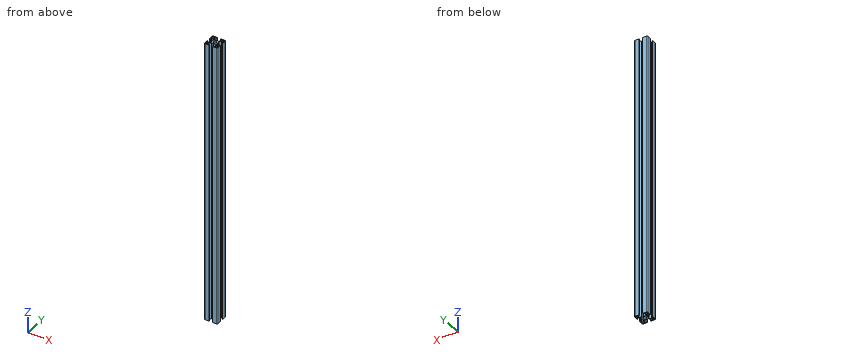
Autodesk Inventor part; units mm, degrees
ref_plane "C1_XY" through (0, 0, 0) normal (0, 0, 1) x (1, 0, 0)
ref_plane "C1_YZ" through (0, 0, 0) normal (1, 0, 0) x (0, 1, 0)
ref_plane "C1_ZX" through (0, 0, 0) normal (0, 1, 0) x (0, 0, 1)
sketch "Sketch_1" plane through (0, 0, 0) normal (0, 0, 1) x (1, 0, 0)
  line L0 (-15, 4) -> (-13, 4)
  line L1 (-13, 4) -> (-13, 8.25)
  line L2 (-13, 8.25) -> (-9.6642, 8.25)
  line L3 (-9.6642, 8.25) -> (-6, 4.5858)
  line L4 (-6, 4.5858) -> (-6, 0.5196)
  line L5 (-6, 0.5196) -> (-5.7, 0)
  line L6 (-5.7, 0) -> (-6, -0.5196)
  line L7 (-6, -0.5196) -> (-6, -4.5858)
  line L8 (-6, -4.5858) -> (-9.6642, -8.25)
  line L9 (-9.6642, -8.25) -> (-13, -8.25)
  line L10 (-13, -8.25) -> (-13, -4)
  line L11 (-13, -4) -> (-15, -4)
  line L12 (-15, -4) -> (-15, -13)
  arc A0 (-15, -13) -> (-13, -15) centre (-13, -13) ccw
  line L13 (-13, -15) -> (-4, -15)
  line L14 (-4, -15) -> (-4, -13)
  line L15 (-4, -13) -> (-8.25, -13)
  line L16 (-8.25, -13) -> (-8.25, -9.6642)
  line L17 (-8.25, -9.6642) -> (-4.5858, -6)
  line L18 (-4.5858, -6) -> (-0.5196, -6)
  line L19 (-0.5196, -6) -> (0, -5.7)
  line L20 (0, -5.7) -> (0.5196, -6)
  line L21 (0.5196, -6) -> (4.5858, -6)
  line L22 (4.5858, -6) -> (8.25, -9.6642)
  line L23 (8.25, -9.6642) -> (8.25, -13)
  line L24 (8.25, -13) -> (4, -13)
  line L25 (4, -13) -> (4, -15)
  line L26 (4, -15) -> (13, -15)
  arc A1 (13, -15) -> (15, -13) centre (13, -13) ccw
  line L27 (15, -13) -> (15, -4)
  line L28 (15, -4) -> (13, -4)
  line L29 (13, -4) -> (13, -8.25)
  line L30 (13, -8.25) -> (9.6642, -8.25)
  line L31 (9.6642, -8.25) -> (6, -4.5858)
  line L32 (6, -4.5858) -> (6, -0.5196)
  line L33 (6, -0.5196) -> (5.7, 0)
  line L34 (5.7, 0) -> (6, 0.5196)
  line L35 (6, 0.5196) -> (6, 4.5858)
  line L36 (6, 4.5858) -> (9.6642, 8.25)
  line L37 (9.6642, 8.25) -> (13, 8.25)
  line L38 (13, 8.25) -> (13, 4)
  line L39 (13, 4) -> (15, 4)
  line L40 (15, 4) -> (15, 13)
  arc A2 (15, 13) -> (13, 15) centre (13, 13) ccw
  line L41 (13, 15) -> (4, 15)
  line L42 (4, 15) -> (4, 13)
  line L43 (4, 13) -> (8.25, 13)
  line L44 (8.25, 13) -> (8.25, 9.6642)
  line L45 (8.25, 9.6642) -> (4.5858, 6)
  line L46 (4.5858, 6) -> (0.5196, 6)
  line L47 (0.5196, 6) -> (0, 5.7)
  line L48 (0, 5.7) -> (-0.5196, 6)
  line L49 (-0.5196, 6) -> (-4.5858, 6)
  line L50 (-4.5858, 6) -> (-8.25, 9.6642)
  line L51 (-8.25, 9.6642) -> (-8.25, 13)
  line L52 (-8.25, 13) -> (-4, 13)
  line L53 (-4, 13) -> (-4, 15)
  line L54 (-4, 15) -> (-13, 15)
  arc A3 (-13, 15) -> (-15, 13) centre (-13, 13) ccw
  line L55 (-15, 13) -> (-15, 4)
extrude "Extrusion1" add sketch "Sketch_1" against normal blind 650
sketch "Sketch2" plane through (0, 0, -650) normal (0, 0, -1) x (-1, 0, 0)
  point P0 (0, 0)
hole "Hole1" at (0, 0, -650) direction (0, 0, 1) diameter 6.8 depth 650
sketch "Sketch3" plane through (0, 0, -650) normal (0, 0, -1) x (-1, 0, 0)
  point P0 (-11.6, 11.6)
hole "Hole2" at (11.6, 11.6, -650) direction (0, 0, 1) diameter 4.2 depth 650
pattern_linear "Rectangular Pattern1" count 2 spacing 23.2 along (-1, 0, 0) count 2 spacing 23.2 along (0, -1, 0) of "Hole2"
ref_plane "C1_XY" through (0, 0, 0) normal (0, 0, 1) x (1, 0, 0)
ref_plane "C1_YZ" through (0, 0, 0) normal (1, 0, 0) x (0, 1, 0)
ref_plane "C1_ZX" through (0, 0, 0) normal (0, 1, 0) x (0, 0, 1)
ref_plane "to_frame_cap1_XY" through (0, 0, 0) normal (0, 0, 1) x (1, 0, 0)
ref_plane "to_frame_cap1_YZ" through (0, 0, 0) normal (1, 0, 0) x (0, 1, 0)
ref_plane "to_frame_cap1_ZX" through (0, 0, 0) normal (0, 1, 0) x (0, 0, 1)
ref_plane "to_frame_cap2_XY" through (0, 0, -650) normal (0, 0, -1) x (1, 0, 0)
ref_plane "to_frame_cap2_YZ" through (0, 0, -650) normal (1, 0, 0) x (0, -1, 0)
ref_plane "to_frame_cap2_ZX" through (0, 0, -650) normal (0, -1, 0) x (0, 0, -1)
properties part number "HFS6-3030-650"
For this review, take the finished solid that the model builds, in its own axes (mm). Round coordinates to 2 decimals unless told otherwise and drop trailing zeros. One line per item, written item: value. Start each with the question number.
Item 1: For L1, parallel to X at y = -4.5, z = -395.5; L2, parallel to Y at x = 11.6, z = -447.5; L3, parallel to X at y = 12.25, z = -338.5, list the stretches that pass through material, from the lowest coordinate up.
Item 2: Clearance check with flat-ended pins moving along their axes: pin 1 Ø2 at (x, z) = (-2.5, -290) entering from -Y; pin 2 Ø0.6 at (y, z) = (13.5, -186.5) entering from -X; pin 3 Ø0.6 at (x, z) = (13.5, -345.5) entering from -Y. State where each tip first meets the part, or that it passes through.
Item 3: Take a section at A-A (z = -437.5). State how many separate pieces and enclosed holes the cut face has, plus the area to 3 significant figures.
Answer below:
1. L1: x = -15 to -13, -6 to 6, 13 to 15
1. L2: y = -15 to -13.7, -9.5 to -8.25, 8.25 to 9.5, 13.7 to 15
1. L3: x = -15 to -13.6, -9.6 to -8.25, 8.25 to 9.6, 13.6 to 15
2. pin 1: stops at y = -6
2. pin 2: stops at x = -14.99
2. pin 3: stops at y = -14.99
3. separate pieces: 1
3. enclosed holes: 5
3. area: 332 mm2
